Geometry: final body of the model. Coordinates: model frame, mm. A direction names the side the tool comes from. Give positions to 0.01 mm unless a question says otherwise; leave off trailing zeros. Write each loop counter-clockwise with the first axis right and the second up, starting at its lowest first coordinate (ties: lowest second). Pieces come first, ordered by that corner, then holes.
Q1. Pin query (flat end, axial travel): pin 1 (1.5 mm diameter, centred on y = -0.5, z = -597, fed in from +X); pin 2 (8 mm diameter, centred on y = 2.5, z = -553, fed in from -X); pin 3 (5 mm diameter, centred on x = -10.5, y = -3.5, fed in from +Z). Return the tip coordinate at first contact, or that it passes through.
Q2. Cut plane A-A on y = -0.75. Return the cut outline in (x, z).
Q3. Cut plane C-C on z = -512.5. Return the cut outline in (x, y).
Q4. Reachability of faces 5 (the face through (80.073, 0.112, -544.507)), 6 (the face through (69, 8, -534)) from +Z, -Z, +X, -X, +Y, -Y: full face, straight path, thin tool, end or side. Return the list, or none.
Q5. Line query: L1, parallel to X at y = 4.25, z = -497; L2, parallel to X at y = -2.5, z = -580.5; L3, parallel to Z at x = -4, y = 7. Output: solid intervals per line, ascending.
Q6. Draft query along X for faces 1 (the face through (69, -8, -534)), 2 (the face through (52.88, 0.11, -589.66)), 3 (the face through (152.67, 0.112, -625.174)), 4 (the face through (82.012, -0.112, -542.217)). Return one class per face: pulls with the +X half, pulls with the -X half, needs draft (parallel to the pull), parting line crosses it, or undercut.
Q7. Cut plane B-B on x = 4. Return the cut outline in (y, z), plus the area to 3 significant figures.
```python
from build123d import *

# Parameters (mm, degrees)
SKETCH2_W = 3
SKETCH2_H = 16


with BuildPart() as part:
    # Sweep1: sweep along a path in Sketch1
    with BuildLine(Plane(origin=(0, 0, 0), x_dir=(1, 0, 0), z_dir=(0, 1, 0))) as sweep1_path:
        Line((-26.227685645, 550.830501906), (128.462333695, 630.052155615))
        ThreePointArc((128.462333695, 630.052155615), (151.645431275, 624.013717264), (148.296942376, 600.292284483))
        Line((148.296942376, 600.292284483), (15.645377126, 488.004107292))
        ThreePointArc((15.645377126, 488.004107292), (-40.52661613, 495.933278247), (-26.227685645, 550.830501906))
    # Sketch2 → Sweep1 (sweep)
    with BuildSketch(Plane(origin=(15.645377126, 0, -488.004107292), x_dir=(0.646091594, 0, 0.763259885), z_dir=(-0.763259885, 0, 0.646091594))):
        Rectangle(SKETCH2_W, SKETCH2_H)
    sweep(path=sweep1_path.line)


solid = part.part
```
Data:
1. pin 1: stops at x = 147.62
1. pin 2: stops at x = -32.07
1. pin 3: stops at z = -477.51
2. outline: (-26.91, -552.17) - (127.78, -631.39) arc R19.5 ccw to (149.27, -599.15) - (16.61, -486.86) arc R39.5 ccw (long way) to start; hole (-25.54, -549.5) - (129.15, -628.72) arc R16.5 ccw to (147.33, -601.44) - (14.68, -489.15) arc R36.5 ccw (long way) to start
3. outline: (-48.15, -8) - (-45.13, -8) - (-45.13, 8) - (-48.15, 8) - close; (42.26, -8) - (46.91, -8) - (46.91, 8) - (42.26, 8) - close
4. face 5: +Y, -Y
4. face 6: +Z, -Z, +X, -X, +Y
5. L1: x = -42.96 to -39.43, 23.95 to 28.59
5. L2: x = 28.41 to 35, 122.59 to 127.24
5. L3: z = -563.9 to -560.53, -480.84 to -477.81
6. face 1: needs draft
6. face 2: undercut
6. face 3: parting line crosses it
6. face 4: pulls with the +X half
7. outline: (-8, -568) - (8, -568) - (8, -564.63) - (-8, -564.63) - close; (-8, -482.87) - (8, -482.87) - (8, -479.68) - (-8, -479.68) - close
7. area: 105 mm2
